```python
from build123d import *

# Parameters (mm, degrees)
SKETCH1_R               = 13.335
BOSS_EXTRUDE1_DEPTH     = 25.4
SKETCH7_R               = 26.67
BOSS_EXTRUDE3_DEPTH     = 31.75
SKETCH10_R              = 13.335
CUT_EXTRUDE1_DEPTH      = 32.75
CUT_EXTRUDE1_DEPTH_BACK = 32.75


with BuildPart() as part:
    # Sketch1 → Boss-Extrude1 (new body, symmetric)
    with BuildSketch(Plane.XY):
        with BuildLine():
            Line((-101.6, 0), (101.6, 0))
            Line((101.6, 0), (101.6, 19.05))
            Line((101.6, 19.05), (45.510728203, 125.565242403))
            ThreePointArc((45.510728203, 125.565242403), (0, 153.035), (-45.510728203, 125.565242403))
            Line((-45.510728203, 125.565242403), (-101.6, 19.05))
            Line((-101.6, 19.05), (-101.6, 0))
        make_face()
        with Locations((0, 101.6)):
            Circle(SKETCH1_R, mode=Mode.SUBTRACT)
    extrude(amount=BOSS_EXTRUDE1_DEPTH, both=True)

    # Sketch7 → Boss-Extrude3 (add, symmetric)
    with BuildSketch(Plane.XY):
        with Locations((0, 101.6)):
            Circle(SKETCH7_R)
    extrude(amount=BOSS_EXTRUDE3_DEPTH, both=True)

    # Sketch10 → Cut-Extrude1 (cut, two sides)
    with BuildSketch(Plane.XY) as cut_extrude1_sk:
        with Locations((0, 101.6)):
            Circle(SKETCH10_R)
    extrude(amount=CUT_EXTRUDE1_DEPTH, mode=Mode.SUBTRACT)
    extrude(cut_extrude1_sk.sketch, amount=-CUT_EXTRUDE1_DEPTH_BACK, mode=Mode.SUBTRACT)


solid = part.part
```
The listing builds one solid part. Answer for the finished solid, in the listing's coordinates (mm). A direction names the side the tool comes from. Round coordinates to 2 decimals unless told otherwise and drop trailing zeros. Loops run counter-clockwise (first coordinate to the right, second up) from the corner with the lowest first, then second, coordinate; pieces in that order, holes last.
Q1. Section B-B, the plane y = 101.6 is taken. Determine the outline of the cut face in (x, z) (3 decimals).
Q2. Which of the six approach directions +Z, -Z, +X, -X, +Y, -Y give full straight-line access (tool end or side, diameter ignored) to faces 5 (the face through (6, 114, -31.75)), 6 (the face through (-3.472, 128.043, 28.619))?
Q3. Given pin 1 Ø3 at (y, z) = (104.5, 14.5) entering from +X; pin 2 Ø3 at (x, y) = (-39.5, 59) entering from -Z; pin 3 Ø4 at (x, z) = (-81, 19.5) entering from +Y, each flat-ended and moving along its own axis, determine where each tip first touches the part or whether it passes through.
Q4. For a pull along Y with two mould halves and no side action, classify faces 1 (the face through (73.95, 71.56, 0.36)), 2 (the face through (-3.472, 128.043, -28.531)), 3 (the face through (6, 114, 31.75)), 4 (the face through (-2.89, 88.58, 0.44)) as released by +Y, released by -Y, zero draft, split by the parting line, or undercut.
Q5. Section A-A, the plane x = 0 is taken. Determine the outline of the cut face in (y, z) (3 decimals), then the cut area to 3 significant figures.
Q6. Find the intervals of material crossed by line 1 (Y direction, x = 0, z = -8) (3 decimals); line 2 (Z direction, x = 22.5, y = 116.5); line 3 (X direction, y = 101.6, z = 19) (3 decimals), in increasing order.
Q7. Section C-C, the plane z = -9.5 is taken. Determine the outline of the cut face in (x, y) (3 decimals), then the cut area to 3 significant figures.
Q8. Section D-D, the plane y = 120 is taken. Determine the outline of the cut face in (x, z), then the cut area to 3 significant figures.
Completed:
1. outline: (-58.13, -25.4) - (-26.67, -25.4) - (-26.67, -31.75) - (-13.335, -31.75) - (-13.335, 31.75) - (-26.67, 31.75) - (-26.67, 25.4) - (-58.13, 25.4) - close; (13.335, -31.75) - (26.67, -31.75) - (26.67, -25.4) - (58.13, -25.4) - (58.13, 25.4) - (26.67, 25.4) - (26.67, 31.75) - (13.335, 31.75) - close
2. face 5: -Z, +X, -X, +Y, -Y
2. face 6: +Z
3. pin 1: stops at x = 57.39
3. pin 2: stops at z = -25.4
3. pin 3: stops at y = 61.97
4. face 1: released by +Y
4. face 2: split by the parting line
4. face 3: zero draft
4. face 4: undercut
5. outline: (0, -25.4) - (74.93, -25.4) - (74.93, -31.75) - (88.265, -31.75) - (88.265, 31.75) - (74.93, 31.75) - (74.93, 25.4) - (0, 25.4) - close; (114.935, -31.75) - (128.27, -31.75) - (128.27, -25.4) - (153.035, -25.4) - (153.035, 25.4) - (128.27, 25.4) - (128.27, 31.75) - (114.935, 31.75) - close
5. area: 6,760 mm2
6. line 1: y = 0 to 88.265, 114.935 to 153.035
6. line 2: z = -25.4 to 25.4
6. line 3: x = -58.13 to -13.335, 13.335 to 58.13
7. outline: (-101.6, 0) - (101.6, 0) - (101.6, 19.05) - (45.511, 125.565) arc R51.435 ccw to (-45.511, 125.565) - (-101.6, 19.05) - close; hole circle Ø26.67 at (0, 101.6)
7. area: 20,800 mm2
8. outline: (-48.44, -25.4) - (-19.31, -25.4) - (-19.31, -31.75) - (19.31, -31.75) - (19.31, -25.4) - (48.44, -25.4) - (48.44, 25.4) - (19.31, 25.4) - (19.31, 31.75) - (-19.31, 31.75) - (-19.31, 25.4) - (-48.44, 25.4) - close
8. area: 5,410 mm2
